Input: part model. Units: mm. Frame: model coordinates. Round coordinates to 2 decimals unless told otherwise and drop trailing zeros. Loops run counter-clockwise (first coordinate to the right, second up) from the corner with the lowest first, then second, coordinate; pieces in that order, holes last. Notation, with made-up numbers: (52.5, 15) -> (70.5, 15) arc R21 cw to (70.5, 22) -> close; hole circle Ø1 at (-9, 34). An arc over 180 degrees is marked (long way). Answer as a JSON object with one key per item and string values. Group by question number.
Item 1: Draft query along Y for faces 1 (the flat face through (11, 11, -89)), 2 (the cylindrical face through (-14.987, -0.624, -88.507)), 3 (the cylindrical face through (13.17, -20.66, -88.51)). Return one class per face: released by +Y, released by -Y, zero draft, split by the parting line, or undercut.
Item 2: Section query A-A on x = 0. Return loops of the section in (y, z).
Item 3: Material intervals for line 1 (X direction, y = -0.5, z = -88.7); line 2 (Y direction, x = 0.5, z = -88.8); line 3 (Y direction, x = -10, z = -88.25), sorted ascending. Write a range as [from, to].
Item 4: Section query C-C on z = -88.65. Return loops of the section in (x, y).
Item 5: Section query D-D on x = 14. Return loops of the section in (y, z).
Item 6: Section query B-B on y = 0. Return loops of the section in (x, z), and give its area (3 significant figures).
Item 7: Pin query (flat end, axial travel): pin 1 (0.5 mm diameter, centred on y = 0.5, z = -88.5, fed in from -X). Return the tip coordinate at first contact, or that it passes through.
from build123d import *

# Parameters (mm, degrees)
SKETCH1_W                    = 9.5
SKETCH1_H                    = 1
SKETCH2_W                    = 2.7
SKETCH2_H                    = 1
EX_INNER_TAB_5MM_M27_5_DEPTH = 2.5


with BuildPart() as part:
    # Sketch1 → REV_MB6_30x49x1 (revolve)
    with BuildSketch(Plane(origin=(0, 0, 0), x_dir=(1, 0, 0), z_dir=(0, 1, 0))):
        with Locations((19.75, 88.5)):
            Rectangle(SKETCH1_W, SKETCH1_H)
    revolve(axis=Axis((0, 0, 150), (0, 0, -1)))

    # Sketch2 → EX_Inner_Tab_5mm_M27.5 (add, symmetric)
    with BuildSketch(Plane(origin=(0, 0, 0), x_dir=(1, 0, 0), z_dir=(0, 1, 0))):
        with Locations((13.85, 88.5)):
            Rectangle(SKETCH2_W, SKETCH2_H)
    extrude(amount=EX_INNER_TAB_5MM_M27_5_DEPTH, both=True)


solid = part.part
Solved:
{
 "1": {"face 1": "zero draft", "face 2": "undercut", "face 3": "split by the parting line"},
 "2": {"outline": "(-24.5, -89) -> (-15, -89) -> (-15, -88) -> (-24.5, -88) -> close; (15, -89) -> (24.5, -89) -> (24.5, -88) -> (15, -88) -> close"},
 "3": {"line 1": "[-24.49, -14.99], [12.5, 24.49]", "line 2": "[-24.49, -14.99], [14.99, 24.49]", "line 3": "[-22.37, -11.18], [11.18, 22.37]"},
 "4": {"outline": "circle Ø49 at (0, 0); hole (12.5, -2.5) -> (12.5, 2.5) -> (14.79, 2.5) arc R15 ccw (long way) to (14.79, -2.5) -> close"},
 "5": {"outline": "(-20.11, -89) -> (-5.39, -89) -> (-5.39, -88) -> (-20.11, -88) -> close; (-2.5, -89) -> (2.5, -89) -> (2.5, -88) -> (-2.5, -88) -> close; (5.39, -89) -> (20.11, -89) -> (20.11, -88) -> (5.39, -88) -> close"},
 "6": {"outline": "(-24.5, -89) -> (-15, -89) -> (-15, -88) -> (-24.5, -88) -> close; (12.5, -89) -> (24.5, -89) -> (24.5, -88) -> (12.5, -88) -> close", "area": "21.5 mm²"},
 "7": {"pin 1": "x = -24.5"}
}
